```python
from build123d import *

# Parameters (mm, degrees)
BOSS_EXTRUDE1_DEPTH = 12.7
SKETCH3_R           = 6.35
CUT_EXTRUDE1_DEPTH  = 74.955735381
FILLET1_R           = 1.27


with BuildPart() as part:
    # Sketch2 → Boss-Extrude1 (new, symmetric)
    with BuildSketch(Plane.XY):
        Polygon((66.675, -2.54), (59.2487587, -26.830140801), (54.39073054, -25.344892541), (61.362885877, -2.54), (-61.362885877, -2.54), (-54.39073054, -25.344892541), (-59.2487587, -26.830140801), (-66.675, -2.54), (-66.675, 2.54), (66.675, 2.54), align=None)
    extrude(amount=BOSS_EXTRUDE1_DEPTH, both=True)

    # Sketch3 → Cut-Extrude1 (cut, through all)
    with BuildSketch(Plane(origin=(0, 2.54, 0), x_dir=(1, 0, 0), z_dir=(0, 1, 0))):
        with Locations(Location((0, 0, 0), (0, 0, 270))):
            Circle(SKETCH3_R)
    extrude(amount=-CUT_EXTRUDE1_DEPTH, mode=Mode.SUBTRACT)

    # Fillet1
    fillet1_edges = [part.edges().sort_by_distance(p)[0] for p in [
        (66.675, -2.54, 0),
        (61.362885877, -2.54, 0),
        (-61.362885877, -2.54, 0),
        (-66.675, -2.54, 0),
        (-66.675, 2.54, 0),
        (66.675, 2.54, 0),
    ]]
    fillet(fillet1_edges, radius=FILLET1_R)


solid = part.part
```
Geometry check sheet. Reference: the model listing, model coordinates, mm. A direction names the side the tool comes from. Round coordinates to 2 decimals unless told otherwise and drop trailing zeros. Loops run counter-clockwise (first coordinate to the right, second up) from the corner with the lowest first, then second, coordinate; pieces in that order, holes last. Notation, with made-up numbers: (53, 11) - (69, 11) arc R8 ccw to (69, 26) - close; hole circle Ø11 at (-19, -37). An arc over 180 degrees is marked (long way). Write each question's results on one line, items separated by ' | '. Start each with the question number.
Q1. Thickness scan on line 1 (X direction, y = -0.6, z = 0) (3 decimals); line 2 (Y direction, x = -11, z = 8.75); line 3 (X direction, y = -23.25, z = 0.5). Record the ranges inside material, lowest first. Write a range as [from, to].
Q2. Gauge pin test, flat ends, axial feed: P1, Ø1.5, axis at y = -16.5, z = -9.5, coming from the +X side; P2, Ø1, axis at y = -22.5, z = -2, coming from the +X side; P3, Ø2, axis at x = 43, z = -2.5, coming from the -Y side. Record the tip position at first contact, or that the pin passes through.
Q3. Access from +Z, -Z, +X, -X, +Y, -Y to the whole of each face (thin tool, end or side, straight path). Record for faces 1 (the flat face through (56.854, -26.098, 0.178)), 2 (the flat face through (-57.671, -14.615, 0.178)), 3 (the flat face through (-66.675, -1, 0)).
Q4. Cross-section at B-B on x = 0. Enter the section's corners in (y, z), and give its area (3 significant figures).
Q5. Cross-section at C-C on y = -5.5. Enter the section's corners in (x, z), and give its area (3 significant figures).
Q6. Release check for a two-part mould opening along Y. For faces 4 (the flat face through (-1, 2.54, 9)), 5 (the flat face through (57.58, -14.91, 0.18)), 6 (the flat face through (-56.79, -26.08, 0.18)), 7 (the flat face through (66.675, -1, 0)) record: +Y half, -Y half, draft (parallel to the pull), parting line (faces both ways), or undercut.
Answers below:
1) line 1: x = [-66.675, -6.35], [6.35, 66.675] | line 2: y = [-2.54, 2.54] | line 3: x = [-60.34, -55.03], [55.03, 60.34]
2) P1: stops at x = 62.64 | P2: stops at x = 60.73 | P3: stops at y = -2.54
3) face 1: +Z, -Z, -Y | face 2: +Z, -Z | face 3: +Z, -Z, -X, +Y, -Y
4) outline: (-2.54, -12.7) - (2.54, -12.7) - (2.54, -6.35) - (-2.54, -6.35) - close; (-2.54, 6.35) - (2.54, 6.35) - (2.54, 12.7) - (-2.54, 12.7) - close | area: 64.5 mm²
5) outline: (-65.77, -12.7) - (-60.46, -12.7) - (-60.46, 12.7) - (-65.77, 12.7) - close; (60.46, -12.7) - (65.77, -12.7) - (65.77, 12.7) - (60.46, 12.7) - close | area: 270 mm²
6) face 4: +Y half | face 5: undercut | face 6: -Y half | face 7: draft
